Geometry: final body of the model. Coordinates: model frame, mm. Face numbers are marked on the shaded views. Give positions to 0.01 mm unless a question says otherwise; leave off trailing zeros. Write each loop counter-clockwise with the first axis right and the second up, starting at its lowest first coordinate (ties: lowest second). Pieces come first, ordered by that corner, then holes. Notation, with made-up numbers: (-18, 19) -> (4, 19) arc R15 cw to (4, 27) -> close; hole circle Ø8 at (12.25, 65). An arc over 180 degrees is marked (long way). Answer as a JSON object with one key per item and string values.
from build123d import *

# Parameters (mm, degrees)
SKETCH7_W                    = 2.54
SKETCH7_H                    = 0.254
F_69_0_0292_DIAMETER_HOLE1_D = 0.74168


with BuildPart() as part:
    # Sweep2: sweep along a path in Sketch1
    with BuildLine(Plane.XY) as sweep2_path:
        Line((-43.18, 0), (-40.64, 0))
        Line((-40.64, 0), (-21.59, 6.35))
        Line((-21.59, 6.35), (-2.54, 0))
        Line((-2.54, 0), (0, 0))
    # Sketch7 → Sweep2 (sweep)
    with BuildSketch(Plane(origin=(0, 0, 0), x_dir=(0, 0, -1), z_dir=(1, 0, 0))):
        with Locations((1.27, 0.127)):
            Rectangle(SKETCH7_W, SKETCH7_H)
    sweep(path=sweep2_path.line, transition=Transition.RIGHT)

    # #69 (0.0292) Diameter Hole1 (through all)
    with Locations(Plane.XZ):
        with Locations((-41.4782, -1.27), (-1.7018, -1.27)):
            Hole(F_69_0_0292_DIAMETER_HOLE1_D / 2)


solid = part.part
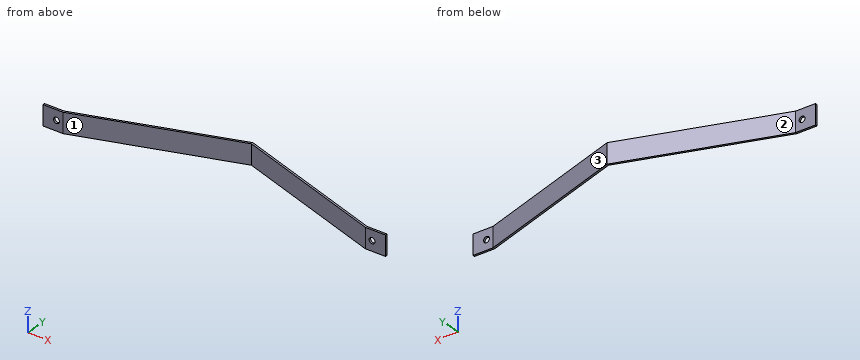
Q1. Cut plane A-A (z = -1.27). Return the cut outline in (x, y), and give its area (3 significant figures).
Values:
{"outline": "(-43.18, 0) -> (-41.85, 0) -> (-41.85, 0.25) -> (-43.18, 0.25) -> close; (-41.11, 0) -> (-40.64, 0) -> (-21.59, 6.35) -> (-2.54, 0) -> (-2.07, 0) -> (-2.07, 0.25) -> (-2.5, 0.25) -> (-21.59, 6.62) -> (-40.68, 0.25) -> (-41.11, 0.25) -> close; (-1.33, 0) -> (0, 0) -> (0, 0.25) -> (-1.33, 0.25) -> close", "area": "11.1 mm²"}
Q2. Cut plane B-B (y = 2.75). Return the cut outline in (x, z), and give its area (3 significant figures).
Values:
{"outline": "(-33.19, -2.54) -> (-32.39, -2.54) -> (-32.39, 0) -> (-33.19, 0) -> close; (-10.79, -2.54) -> (-9.99, -2.54) -> (-9.99, 0) -> (-10.79, 0) -> close", "area": "4.08 mm²"}
Q3. Cut plane C-C (x = -3). Return the cut outline in (y, z), and give its area (3 significant figures).
Values:
{"outline": "(0.15, -2.54) -> (0.42, -2.54) -> (0.42, 0) -> (0.15, 0) -> close", "area": "0.680 mm²"}
Q4. Mould query, pull axis X, two halves, no side actions, for the marked faces 1, 2 and 3. Classes: pulls with the +X half, pulls with the -X half, needs draft (parallel to the pull), parting line crosses it, or undercut.
Values:
{"face 1": "undercut", "face 2": "pulls with the -X half", "face 3": "pulls with the +X half"}
Q5. Material intervals for L1, parallel to Y at x = -18, z = -1.2; L2, parallel to Y at x = -9, z = -0.95, sorted ascending. Write a range as from..to.
Values:
{"L1": "5.15..5.42", "L2": "2.15..2.42"}
